```python
from build123d import *

# Parameters (mm, degrees)
F1_DEPTH = 10


with BuildPart() as f1:
    # F0 (on Top) → F1 (new body)
    with BuildSketch(Plane.XY):
        Polygon((3.464102, 6), (-3.464102, 6), (-6.928203, 0), (-3.464102, -6), (3.464102, -6), (6.928203, 0), align=None)
        with BuildLine():
            ThreePointArc((-0.54173, -4.769332), (-3.218595, -3.560989), (-4.690485, -1.019485))
            ThreePointArc((-4.690485, -1.019485), (-3.432213, -2.356022), (-1.630911, -2.709417))
            ThreePointArc((-1.630911, -2.709417), (-1.417251, -3.914354), (-0.54173, -4.769332))
        make_face(mode=Mode.SUBTRACT)
        with BuildLine():
            Line((1.986308, 0.885414), (0.209216, 1.704124))
            ThreePointArc((0.209216, 1.704124), (-0.454124, 1.459216), (-0.209216, 0.795876))
            Line((-0.209216, 0.795876), (1.593748, -0.034753))
            ThreePointArc((1.593748, -0.034753), (2.75641, -1.894851), (1.51377, -3.702499))
            ThreePointArc((1.51377, -3.702499), (1.000033, -3.872975), (0.467983, -3.97253))
            ThreePointArc((0.467983, -3.97253), (-0.580071, -3.344267), (-0.237933, -2.171206))
            ThreePointArc((-0.237933, -2.171206), (-0.232163, -2.167033), (-0.226363, -2.162901))
            Line((-0.226363, -2.162901), (1.371207, -1.033248))
            ThreePointArc((1.371207, -1.033248), (1.49078, -0.336325), (0.793857, -0.216752))
            Line((0.793857, -0.216752), (-0.826971, -1.36285))
            ThreePointArc((-0.826971, -1.36285), (-3.019194, -1.439695), (-3.963343, 0.540286))
            ThreePointArc((-3.963343, 0.540286), (-3.854111, 1.070434), (-3.674303, 1.580979))
            ThreePointArc((-3.674303, 1.580979), (-2.599148, 2.1734), (-1.759946, 1.277486))
            Line((-1.759946, 1.277486), (-1.580423, -0.670876))
            ThreePointArc((-1.580423, -0.670876), (-1.036656, -1.122891), (-0.584641, -0.579124))
            Line((-0.584641, -0.579124), (-0.766777, 1.397603))
            ThreePointArc((-0.766777, 1.397603), (0.262784, 3.334546), (2.449573, 3.162213))
            ThreePointArc((2.449573, 3.162213), (2.854078, 2.802541), (3.20632, 2.39155))
            ThreePointArc((3.20632, 2.39155), (3.186256, 1.169777), (1.999286, 0.879547))
            ThreePointArc((1.999286, 0.879547), (1.992787, 0.882458), (1.986308, 0.885414))
        make_face(mode=Mode.SUBTRACT)
        with BuildLine():
            ThreePointArc((3.228143, -3.552336), (3.756481, -1.794373), (3.161879, -0.057702))
            ThreePointArc((3.161879, -0.057702), (4.098556, 0.729802), (4.401228, 1.915514))
            ThreePointArc((4.401228, 1.915514), (4.693205, -1.006891), (3.228143, -3.552336))
        make_face(mode=Mode.SUBTRACT)
        with BuildLine():
            ThreePointArc((-3.859498, 2.853818), (-1.474328, 4.567971), (1.462906, 4.571641))
            ThreePointArc((1.462906, 4.571641), (-0.323966, 4.150419), (-1.530858, 2.767033))
            ThreePointArc((-1.530858, 2.767033), (-2.681235, 3.18455), (-3.859498, 2.853818))
        make_face(mode=Mode.SUBTRACT)
    extrude(amount=F1_DEPTH)


solid = f1.part
```
Geometry: final body of the model. Coordinates: model frame, mm. A direction names the side the tool comes from. Give positions to 0.01 mm unless a question says otherwise; leave off trailing zeros. Loops run counter-clockwise (first coordinate to the right, second up) from the corner with the lowest first, then second, coordinate; pieces in that order, holes last. Notation, with made-up numbers: (63, 10.25) -> (71, 10.25) arc R17 cw to (71, 27.25) -> close; hole circle Ø10 at (-21, 24.5). An arc over 180 degrees is marked (long way). Use CSV: the item, a comma, the result in double quotes.
(1) First-contact query: P1, Ø5, axis at x = 3.5, z = 8, coming from the -Y side; P2, Ø3, axis at y = 4, z = 5, coming from the -X side; P3, Ø3, axis at x = 5.5, z = 3, coming from the -Y side. Flat tips, straight axial feed; report the tip coordinate or a pass-through.
From the geometry:
P1,"y = -6"
P2,"x = -5.48"
P3,"y = -5.07"
(2) Cut plane A-A (x = 1). Output: boundary loops of the cut face in (y, z), plus the area to 3 significant figures.
From the geometry:
outline,"(-6, 0) -> (-3.87, 0) -> (-3.87, 10) -> (-6, 10) -> close; (-1.3, 0) -> (-0.13, 0) -> (-0.13, 10) -> (-1.3, 10) -> close; (0.24, 0) -> (1.34, 0) -> (1.34, 10) -> (0.24, 10) -> close; (3.57, 0) -> (4.57, 0) -> (4.57, 10) -> (3.57, 10) -> close; (4.69, 0) -> (6, 0) -> (6, 10) -> (4.69, 10) -> close"
area,"67.0 mm^2"
(3) Cut plane C-C (z = 3.75). Count the separate pieces of the cut face and the enclosed holes in it, plus the area to 3 significant figures.
From the geometry:
separate pieces,"1"
enclosed holes,"4"
area,"87.5 mm^2"
(4) Access query for faces 1 (the face through (-3.856, 1.063, 4.93)), 2 (the face through (0, 1, 10)). Directions: +Z, -Z, +X, -X, +Y, -Y. A direction counts if a zero-diameter tool reaches every point of the face in a straight line with its end or side. Return the directions, or none.
From the geometry:
face 1,"+Z, -Z"
face 2,"+Z, +X, -X, +Y, -Y"
(5) Ray query, line 1 along Y through (x, z) = (-1.25, 3.75); line 2 along X through (y, z) = (0.5, 1.5); line 3 along Y through (x, z) = (-1, 1). Return the intervals inside material, ascending. Write a range as [from, to].
From the geometry:
line 1,"[-6, -4.63], [-4.18, -1.59], [-1.1, 3.28], [4.63, 6]"
line 2,"[-6.64, -3.97], [-1.69, -0.68], [0.43, 3.93], [4.77, 6.64]"
line 3,"[-6, -4.69], [-4.45, -1.47], [-1.12, 3.59], [4.69, 6]"
(6) Pull-direction query (X, two-part tool) for faces 3 (the face through (5.172, -3.042, 4.93)), 4 (the face through (0, 6, 5)), 5 (the face through (3.757, -1.82, 4.93)); classes: released by +X, released by -X, zero draft, split by the parting line, or undercut.
From the geometry:
face 3,"released by +X"
face 4,"zero draft"
face 5,"undercut"
(7) Cut plane B-B (y = 5). Output: boundary loops of the cut face in (x, z), plus the area to 3 significant figures.
From the geometry:
outline,"(-4.04, 0) -> (4.04, 0) -> (4.04, 10) -> (-4.04, 10) -> close"
area,"80.8 mm^2"
